```python
from build123d import *

# Parameters (mm, degrees)
BOSS_EXTRUDE1_DEPTH = 10
M4_TAPPED_HOLE1_D   = 3.3
M8_TAPPED_HOLE1_D   = 6.8


with BuildPart() as part:
    # Sketch1 → Boss-Extrude1 (new body)
    with BuildSketch(Plane.XY):
        Polygon((-80, 39), (80, 39), (80, 29), (90, 29), (90, -29), (80, -29), (80, -39), (-80, -39), (-80, -29), (-90, -29), (-90, 29), (-80, 29), align=None)
    extrude(amount=BOSS_EXTRUDE1_DEPTH)

    # M4 Tapped Hole1 (through all)
    with Locations(Plane.XY.offset(10)):
        with Locations((-68, 30.75), (-68, -30.75), (68, -30.75), (68, 30.75)):
            Hole(M4_TAPPED_HOLE1_D / 2)

    # M8 Tapped Hole1 (through all)
    with Locations(Plane.XY.offset(10)):
        with Locations((-59, 30.5), (-59, -30.5), (59, -30.5), (59, 30.5)):
            Hole(M8_TAPPED_HOLE1_D / 2)


solid = part.part
```
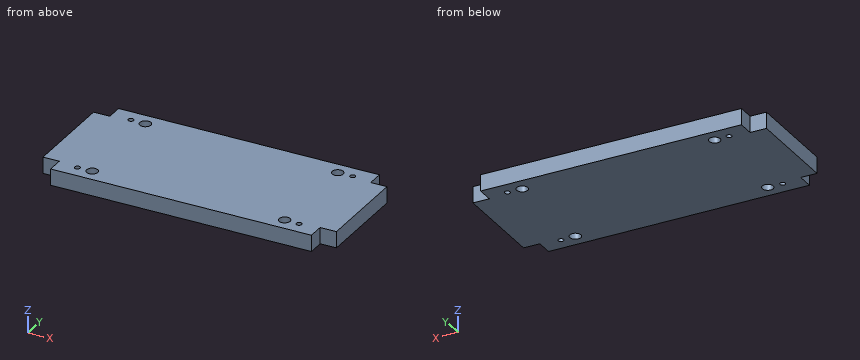
Geometry: final body of the model. Coordinates: model frame, mm. Coordinates: 2 decimals unless noted, no trailing zeros. Order: outer loops, then holes, each group sorted by start corner. A loop starts at its lowest first (then second) coordinate and runs counter-clockwise, first axis right, second up. Notation, with made-up numbers: (78.25, 36) -> (109.25, 36) arc R20 ccw to (109.25, 49) -> close; hole circle Ø1 at (67, -11). An arc over 180 degrees is marked (long way). Use CSV: the item, a comma, the result in double quotes.
1) Section C-C on x = -59. Output: boundary loops of the cut face in (y, z), then the cut area to 3 significant figures.
Findings:
outline,"(-39, 0) -> (-33.9, 0) -> (-33.9, 10) -> (-39, 10) -> close; (-27.1, 0) -> (27.1, 0) -> (27.1, 10) -> (-27.1, 10) -> close; (33.9, 0) -> (39, 0) -> (39, 10) -> (33.9, 10) -> close"
area,"644 mm^2"
2) Section B-B on x = 68. Output: boundary loops of the cut face in (y, z).
Findings:
outline,"(-39, 0) -> (-32.4, 0) -> (-32.4, 10) -> (-39, 10) -> close; (-29.1, 0) -> (29.1, 0) -> (29.1, 10) -> (-29.1, 10) -> close; (32.4, 0) -> (39, 0) -> (39, 10) -> (32.4, 10) -> close"
3) Section A-A on z = 6.75. State how many separate pieces and enclosed holes the cut face has, then the cut area to 3 significant figures.
Findings:
separate pieces,"1"
enclosed holes,"8"
area,"13,500 mm^2"
4) Pin query (flat end, axial travel): pin 1 Ø5 at (y, z) = (36.5, 2.5) entering from +X; pin 2 Ø5 at (x, z) = (84, 7) entering from -Y; pin 3 Ø5 at (y, z) = (-35, 5.5) entering from -X. Return the tip coordinate at first contact, or that it passes through.
Findings:
pin 1,"stops at x = 80"
pin 2,"stops at y = -29"
pin 3,"stops at x = -80"
5) Line query: line 1 (Y direction, x = 59, z = 8.25); line 2 (Y direction, x = 68, z = 5.25). Output: solid intervals per line, ascending.
Findings:
line 1,"y = -39 to -33.9, -27.1 to 27.1, 33.9 to 39"
line 2,"y = -39 to -32.4, -29.1 to 29.1, 32.4 to 39"
